Part model, mm, in its own coordinate system. Face numbers are marked on the shaded views. A direction names the side the tool comes from. Round coordinates to 2 decimals unless told otherwise and drop trailing zeros. Loops run counter-clockwise (first coordinate to the right, second up) from the corner with the lowest first, then second, coordinate; pieces in that order, holes last.
(1) Cut at D-D on x = -29.5. List the corners of the cut face in (y, z).
(2) Mould opens along X. For the marked faces 1, 2 and 3 say: +X half, -X half, draft (parallel to the pull), parting line (faces both ways), or undercut.
(3) Tool access for the marked faces 4, 5, 6 and 7: list every direction of +Z, -Z, +X, -X, +Y, -Y with a clear straight run to the whole face (end or side of a thin tool).
(4) Cut at C-C on y = -12. List the corners of the cut face in (x, z).
(5) Flat gauge pins, fed straight in: pin 1 (1 mm diameter, centred on x = -22, y = -34, fed in from +Z); pin 2 (9.5 mm diameter, centred on y = -16.5, z = 17, fed in from +X); pin 3 (5 mm diameter, centred on y = -0.5, z = 16.5, fed in from -X). Where does each tip first touch, or does it go through?
(6) Cut at A-A on z = 13.75. List the corners of the cut face in (x, y).
(7) Probe probe 1 along Y at (x, z) = (52, 11.75); probe 2 along Y at (x, z) = (1.5, 5.75); probe 3 along Y at (x, z) = (-8, 2). List the from-to ranges inside material, lowest first.
(8) Cut at B-B on x = 19. List the corners of the cut face in (y, z), then the cut area to 3 significant figures.
from build123d import *

# Parameters (mm, degrees)
F0_W     = 74.6637145057
F0_H     = 23.7817782909
F0_W_2   = 58.2561278716
F0_H_2   = 9.5864515752
F1_DEPTH = 25.4
F2_T     = -2.54


with BuildPart() as f1:
    # F0 (on Top) → F1 (new body)
    with BuildSketch(Plane.XY):
        Polygon((60.7449188828, 55.3986318409), (-37.3318567872, 55.3986318409), (-37.3318567872, 27.7454033494), (-37.1474996209, 27.7454033494), (-10.6004038826, 27.7454033494), (60.7449188828, 27.7454033494), align=None)
        Polygon((-10.6004038826, 27.7454033494), (-37.1474996209, 27.7454033494), (-37.1474996209, -47.4713742733), (-10.6004038826, -47.4713742733), (-10.6004038826, -23.6895959824), (-10.6004038826, -4.8854034394), (-10.6004038826, 4.7010481358), align=None)
        with Locations((26.7314533703, -35.5804851279)):
            Rectangle(F0_W, F0_H)
        with Locations((18.5276600532, -0.0921776518)):
            Rectangle(F0_W_2, F0_H_2)
    extrude(amount=F1_DEPTH)

    # F2
    f2_openings = [f1.faces().sort_by_distance(p)[0] for p in [
        (5.947866, 4.234734, 25.4),
    ]]
    offset(amount=F2_T, openings=f2_openings, kind=Kind.INTERSECTION)


solid = f1.part
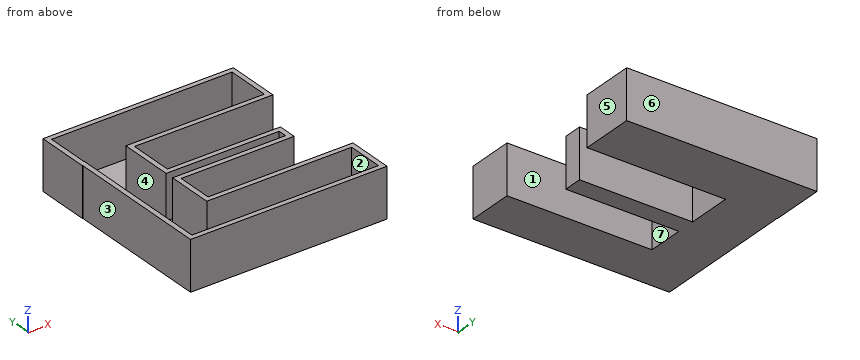
Final values:
1. outline: (-47.47, 0) - (55.4, 0) - (55.4, 25.4) - (52.86, 25.4) - (52.86, 2.54) - (-44.93, 2.54) - (-44.93, 25.4) - (-47.47, 25.4) - close
2. face 1: draft
2. face 2: undercut
2. face 3: -X half
3. face 4: +Z
3. face 5: +Z, -Z, +X, +Y
3. face 6: +Z, -Z, +X, -X, +Y
3. face 7: +Z, -Z, +X
4. outline: (-37.15, 0) - (-10.6, 0) - (-10.6, 25.4) - (-13.14, 25.4) - (-13.14, 2.54) - (-34.61, 2.54) - (-34.61, 25.4) - (-37.15, 25.4) - close
5. pin 1: stops at z = 2.54
5. pin 2: stops at x = -10.6
5. pin 3: stops at x = -37.15
6. outline: (-37.33, 27.75) - (-37.15, 27.75) - (-37.15, -47.47) - (64.06, -47.47) - (64.06, -23.69) - (-10.6, -23.69) - (-10.6, -4.89) - (47.66, -4.89) - (47.66, 4.7) - (-10.6, 4.7) - (-10.6, 27.75) - (60.74, 27.75) - (60.74, 55.4) - (-37.33, 55.4) - close; hole (-34.79, 30.29) - (-34.61, 30.29) - (-34.61, -44.93) - (61.52, -44.93) - (61.52, -26.23) - (-13.14, -26.23) - (-13.14, -2.35) - (45.12, -2.35) - (45.12, 2.16) - (-13.14, 2.16) - (-13.14, 30.29) - (58.2, 30.29) - (58.2, 52.86) - (-34.79, 52.86) - close
7. probe 1: y = -47.47 to -44.93, -26.23 to -23.69, 27.75 to 30.29, 52.86 to 55.4
7. probe 2: y = -47.47 to -44.93, -26.23 to -23.69, -4.89 to -2.35, 2.16 to 4.7, 27.75 to 30.29, 52.86 to 55.4
7. probe 3: y = -47.47 to -23.69, -4.89 to 4.7, 27.75 to 55.4
8. outline: (-47.47, 0) - (-23.69, 0) - (-23.69, 25.4) - (-26.23, 25.4) - (-26.23, 2.54) - (-44.93, 2.54) - (-44.93, 25.4) - (-47.47, 25.4) - close; (-4.89, 0) - (4.7, 0) - (4.7, 25.4) - (2.16, 25.4) - (2.16, 2.54) - (-2.35, 2.54) - (-2.35, 25.4) - (-4.89, 25.4) - close; (27.75, 0) - (55.4, 0) - (55.4, 25.4) - (52.86, 25.4) - (52.86, 2.54) - (30.29, 2.54) - (30.29, 25.4) - (27.75, 25.4) - close
8. area: 503 mm2
